```python
from build123d import *

# Parameters (mm, degrees)
SKETCH1_W           = 25
SKETCH1_H           = 25
SKETCH1_W_2         = 23
SKETCH1_H_2         = 23
BOSS_EXTRUDE1_DEPTH = 180
CUT_EXTRUDE1_DEPTH  = 183.157212319
CUT_EXTRUDE2_REACH  = 184.157
SKETCH3_R           = 2


with BuildPart() as part:
    # Sketch1 → Boss-Extrude1 (new body)
    with BuildSketch(Plane.XY):
        Rectangle(SKETCH1_W, SKETCH1_H)
        Rectangle(SKETCH1_W_2, SKETCH1_H_2, mode=Mode.SUBTRACT)
    extrude(amount=BOSS_EXTRUDE1_DEPTH)

    # Sketch2 → Cut-Extrude1 (cut, through all)
    with BuildSketch(Plane(origin=(12.5, 0, 0), x_dir=(0, 0, -1), z_dir=(1, 0, 0))):
        Polygon((-180, -12.5), (-165.56624327, 12.5), (-180, 12.5), align=None)
    extrude(amount=-CUT_EXTRUDE1_DEPTH, mode=Mode.SUBTRACT)

    # Sketch3 → Cut-Extrude2 (cut, up to next)
    with BuildSketch(Plane(origin=(0, 12.5, 0), x_dir=(1, 0, 0), z_dir=(0, 1, 0)), mode=Mode.PRIVATE) as cut_extrude2_sk1:
        with Locations(Location((0, -8.5, 0), (0, 0, 270))):
            Circle(SKETCH3_R)
    cut_extrude2_tool1 = extrude(cut_extrude2_sk1.sketch, amount=-CUT_EXTRUDE2_REACH, mode=Mode.PRIVATE) & part.part
    # Sketch3 → Cut-Extrude2 (cut, up to next)
    with BuildSketch(Plane(origin=(0, 12.5, 0), x_dir=(1, 0, 0), z_dir=(0, 1, 0)), mode=Mode.PRIVATE) as cut_extrude2_sk2:
        with Locations(Location((0, -38.5, 0), (0, 0, 270))):
            Circle(SKETCH3_R)
    cut_extrude2_tool2 = extrude(cut_extrude2_sk2.sketch, amount=-CUT_EXTRUDE2_REACH, mode=Mode.PRIVATE) & part.part
    # Sketch3 → Cut-Extrude2 (cut, up to next)
    with BuildSketch(Plane(origin=(0, 12.5, 0), x_dir=(1, 0, 0), z_dir=(0, 1, 0)), mode=Mode.PRIVATE) as cut_extrude2_sk3:
        with Locations(Location((0, -68.5, 0), (0, 0, 270))):
            Circle(SKETCH3_R)
    cut_extrude2_tool3 = extrude(cut_extrude2_sk3.sketch, amount=-CUT_EXTRUDE2_REACH, mode=Mode.PRIVATE) & part.part
    add(cut_extrude2_tool1.solids().sort_by_distance((0, 12.5, 8.5))[0], mode=Mode.SUBTRACT)
    add(cut_extrude2_tool2.solids().sort_by_distance((0, 12.5, 38.5))[0], mode=Mode.SUBTRACT)
    add(cut_extrude2_tool3.solids().sort_by_distance((0, 12.5, 68.5))[0], mode=Mode.SUBTRACT)


solid = part.part
```
Input: part model. Units: mm. Frame: model coordinates. A direction names the side the tool comes from. Give positions to 0.01 mm unless a question says otherwise; leave off trailing zeros. Order: outer loops, then holes, each group sorted by start corner. A loop starts at its lowest first (then second) coordinate and runs counter-clockwise, first axis right, second up. Notation, with made-up numbers: M 78.5,-29 L 116.5,-29 A20 cw 116.5,-24 Z; hole C 79.5,-15 d9. An arc over 180 degrees is marked long. Return JSON: item names as keys, results as strings.
Item 1: Cut plane D-D (z = 38.5). Return loops of the section in (x, y), then the cut area to 3 significant figures.
Solutions:
{"outline": "M -12.5,-12.5 L 12.5,-12.5 L 12.5,12.5 L 2,12.5 L 2,11.5 L 11.5,11.5 L 11.5,-11.5 L -11.5,-11.5 L -11.5,11.5 L -2,11.5 L -2,12.5 L -12.5,12.5 Z", "area": "92.0 mm^2"}
Item 2: First-contact query: P1, Ø12, axis at x = 6, y = -3, coming from the +Z side; P2, Ø2.5, axis at x = 0, z = 8.5, coming from the +Y side; P3, Ø8, axis at x = -0.5, y = -8, coming from the +Z side. Flat tips, straight axial feed; report the tip coordinate or a pass-through.
Solutions:
{"P1": "z = 175.9", "P2": "y = -11.5", "P3": "z = 179.71"}
Item 3: Pull-direction query (Y, two-part tool) for faces 1 (the flat face through (-11.98, -0.98, 173.35)), 2 (the flat face through (11.5, 0, 88)), 3 (the flat face through (-1, -12, 0)); classes: +Y half, -Y half, draft (parallel to the pull), parting line (faces both ways), or undercut.
Solutions:
{"face 1": "+Y half", "face 2": "undercut", "face 3": "draft"}
Item 4: Cut plane A-A (x = 0). Return loops of the section in (y, z).
Solutions:
{"outline": "M -12.5,0 L -11.5,0 L -11.5,179.42 L -12.5,180 Z; M 11.5,0 L 12.5,0 L 12.5,6.5 L 11.5,6.5 Z; M 11.5,10.5 L 12.5,10.5 L 12.5,36.5 L 11.5,36.5 Z; M 11.5,40.5 L 12.5,40.5 L 12.5,66.5 L 11.5,66.5 Z; M 11.5,70.5 L 12.5,70.5 L 12.5,165.57 L 11.5,166.14 Z"}
Item 5: Cut plane C-C (z = 160.5). Return loops of the section in (x, y), then the cut area to 3 significant figures.
Solutions:
{"outline": "M -12.5,-12.5 L 12.5,-12.5 L 12.5,12.5 L -12.5,12.5 Z; hole M -11.5,-11.5 L 11.5,-11.5 L 11.5,11.5 L -11.5,11.5 Z", "area": "96.0 mm^2"}
Item 6: Access query for faces 4 (the flat face through (0, 11.5, 82)), 5 (the flat face through (-12.5, 0, 89)), 6 (the cylindrical face through (0.088, 12.007, 36.502)). Directions: +Z, -Z, +X, -X, +Y, -Y. A direction counts if a zero-diameter tool reaches every point of the face in a straight line with its end or side. Return the directions, or none.
Solutions:
{"face 4": "+Z, -Z", "face 5": "+Z, -Z, -X, +Y, -Y", "face 6": "+Y"}
Item 7: Cut plane B-B (y = 0.5). Return loops of the section in (x, z), then the cut area to 3 significant figures.
Solutions:
{"outline": "M -12.5,0 L -11.5,0 L -11.5,172.49 L -12.5,172.49 Z; M 11.5,0 L 12.5,0 L 12.5,172.49 L 11.5,172.49 Z", "area": "345 mm^2"}
Item 8: Ray query, probe 1 along X at (y, z) = (11.9, 68.5); probe 2 along X at (y, z) = (-11, 129). Return the intervals inside material, ascending.
Solutions:
{"probe 1": "-12.5 to -2, 2 to 12.5", "probe 2": "-12.5 to -11.5, 11.5 to 12.5"}
